For this review, take the finished solid that the model builds, in its own axes (mm). A direction names the side the tool comes from. Give positions to 0.01 mm unless a question says otherwise; leave off trailing zeros. Order: outer loops, then holes, each group sorted by start corner. A loop starts at its lowest first (then second) coordinate and runs counter-clockwise, first axis right, second up. Notation, with made-up numbers: (-1, 30.5) -> (24, 30.5) arc R14 ccw to (24, 37.5) -> close; hole circle Ø5 at (38.25, 0). An arc over 180 degrees is marked (long way). Return JSON: item names as keys, results as strings. Group by question number.
1) Add section A-A (y = -8.25). State how many separate pieces and enclosed holes the cut face has, then the cut area to 3 significant figures.
2) For faces 4 (the face through (19.212, -9.658, 29.498)), 5 (the face through (32.58, -9.66, 33.21)), 6 (the face through (-23.207, -9, 7)), list the 3-axis set-ups (+Z, -Z, +X, -X, +Y, -Y) from which the entire face can be reached by the end or side of a thin tool; tool diameter is ignored.
3) Add section B-B (x = 34). Give the boundary of the cut face in (y, z).
4) The part is to be moulded in two halves that separate along X. For faces 1 (the face through (49.45, -9.33, 42.95)), 2 (the face through (54.58, -9, 43)), 3 (the face through (3, -19.05, 7)), say which applies: released by +X, released by -X, zero draft, split by the parting line, or undercut.
5) Add section D-D (z = 23.5). Give the boundary of the cut face in (x, y), then the cut area to 3 significant figures.
6) Add section C-C (y = -17.5). Give the boundary of the cut face in (x, z).
7) To check wall thickness, follow line 1 along Z through (x, y) = (-38, -16.5); line 2 along Z through (x, y) = (21, -7.5); line 3 along X through (y, z) = (-6.75, -34). State the ranges of each line that lie inside material, in increasing order.
8) Insertion check: P1, Ø5.5, axis at x = -13.68, z = 25.59, coming from the -Y side; P2, Ø10, axis at x = -37.49, y = -9.52, coming from the -Z side; P3, Ø9.5, axis at y = -8.5, z = -4.5, coming from the +X side; P4, Ø5.5, axis at y = -7.5, z = -1, coming from the -X side. Each pin has a flat end and moves straight along its axis. Give the tip position at first contact, or say it passes through.
from build123d import *

# Parameters (mm, degrees)
F1_DEPTH = 19.05
F2_R     = 6.35
F4_D     = 8.8
F5_D     = 8.8


with BuildPart() as f1:
    # F0 (on Front) → F1 (new body)
    with BuildSketch(Plane.XZ):
        Polygon((3.7801079915, 50.9944110171), (-47.0198920085, 50.9944110171), (-47.0198920085, 35.1194110171), (-23.2073920085, 35.1194110171), (-23.2073920085, 6.5444110171), (-23.2073920085, -22.0305889829), (-47.0198920085, -22.0305889829), (-47.0198920085, -37.9055889829), (54.5801079915, -37.9055889829), (54.5801079915, -22.0305889829), (30.7676079915, -22.0305889829), (30.7676079915, 6.5444110171), (30.7676079915, 35.1194110171), (54.5801079915, 35.1194110171), (54.5801079915, 50.9944110171), align=None)
    extrude(amount=F1_DEPTH)

    # F2
    f2_edges = [f1.edges().sort_by_distance(p)[0] for p in [
        (30.767608, -9.525, -22.030589),
        (30.767608, -9.525, 35.119411),
        (-23.207392, -9.525, -22.030589),
        (-23.207392, -9.525, 35.119411),
    ]]
    fillet(f2_edges, radius=F2_R)

    # F4 (through all)
    with Locations(Plane.XY.offset(50.9944110171)):
        with Locations((-37.4948920085, -9.525), (45.0551079915, -9.525)):
            Hole(F4_D / 2)

    # F5 (through all)
    with Locations(Plane(origin=(0, 0, 0), x_dir=(1, 0, 0), z_dir=(0, 1, 0))):
        with Locations((-13.6823920085, -25.5944110171), (21.2426079915, -25.5944110171)):
            Hole(F5_D / 2)


solid = f1.part
Evaluation:
{
 "1": {"separate pieces": "5", "enclosed holes": "2", "area": "5,690 mm^2"},
 "2": {"face 4": "+Y, -Y", "face 5": "+X, +Y, -Y", "face 6": "-X, +Y, -Y"},
 "3": {"outline": "(-19.05, -37.91) -> (0, -37.91) -> (0, -21.21) -> (-19.05, -21.21) -> close; (-19.05, 34.3) -> (0, 34.3) -> (0, 50.99) -> (-19.05, 50.99) -> close"},
 "4": {"face 1": "undercut", "face 2": "released by +X", "face 3": "zero draft"},
 "5": {"outline": "(-23.21, -19.05) -> (-17.55, -19.05) -> (-17.55, 0) -> (-23.21, 0) -> close; (-9.81, -19.05) -> (17.37, -19.05) -> (17.37, 0) -> (-9.81, 0) -> close; (25.11, -19.05) -> (30.77, -19.05) -> (30.77, 0) -> (25.11, 0) -> close", "area": "733 mm^2"},
 "6": {"outline": "(-47.02, -37.91) -> (54.58, -37.91) -> (54.58, -22.03) -> (37.12, -22.03) arc R6.35 cw to (30.77, -15.68) -> (30.77, 28.77) arc R6.35 cw to (37.12, 35.12) -> (54.58, 35.12) -> (54.58, 50.99) -> (-47.02, 50.99) -> (-47.02, 35.12) -> (-29.56, 35.12) arc R6.35 cw to (-23.21, 28.77) -> (-23.21, -15.68) arc R6.35 cw to (-29.56, -22.03) -> (-47.02, -22.03) -> close; hole circle Ø8.8 at (-13.68, 25.59); hole circle Ø8.8 at (21.24, 25.59)"},
 "7": {"line 1": "-37.91 to -22.03, 35.12 to 50.99", "line 2": "-37.91 to 21.2, 29.99 to 50.99", "line 3": "-47.02 to -40.91, -34.08 to 41.64, 48.47 to 54.58"},
 "8": {"P1": "through", "P2": "z = -37.91", "P3": "x = 30.77", "P4": "x = -23.21"}
}
